from build123d import *

# Parameters (mm, degrees)
SKETCH1_R           = 6.35
BOSS_EXTRUDE1_DEPTH = 6.985
SKETCH3_R           = 8.382
BOSS_EXTRUDE2_DEPTH = 3.81
SKETCH5_R           = 2.5527
CUT_EXTRUDE2_DEPTH  = 56.328875207
SKETCH6_R           = 7.747
SKETCH6_R_2         = 6.096
CUT_EXTRUDE3_DEPTH  = 1.27


with BuildPart() as part:
    # Sketch1 → Boss-Extrude1 (new body)
    with BuildSketch(Plane.XY):
        with Locations((43.174261814, 8.550344032)):
            Circle(SKETCH1_R)
    extrude(amount=-BOSS_EXTRUDE1_DEPTH)

    # Sketch3 → Boss-Extrude2 (add)
    with BuildSketch(Plane.XY):
        with Locations(Location((43.174261814, 8.550344032, 0), (0, 0, 180))):
            Circle(SKETCH3_R)
    extrude(amount=BOSS_EXTRUDE2_DEPTH)

    # Sketch5 → Cut-Extrude2 (cut, through all)
    with BuildSketch(Plane(origin=(0, 0, -6.985), x_dir=(-1, 0, 0), z_dir=(0, 0, -1))):
        with Locations(Location((-43.174261814, 8.550344032, 0), (0, 0, 90))):
            Circle(SKETCH5_R)
    extrude(amount=-CUT_EXTRUDE2_DEPTH, mode=Mode.SUBTRACT)

    # Sketch6 → Cut-Extrude3 (cut)
    with BuildSketch(Plane.XY.offset(3.81)):
        with Locations((43.174261814, 8.550344032)):
            Circle(SKETCH6_R)
        with Locations((43.174261814, 8.550344032)):
            Circle(SKETCH6_R_2, mode=Mode.SUBTRACT)
    extrude(amount=-CUT_EXTRUDE3_DEPTH, mode=Mode.SUBTRACT)


solid = part.part
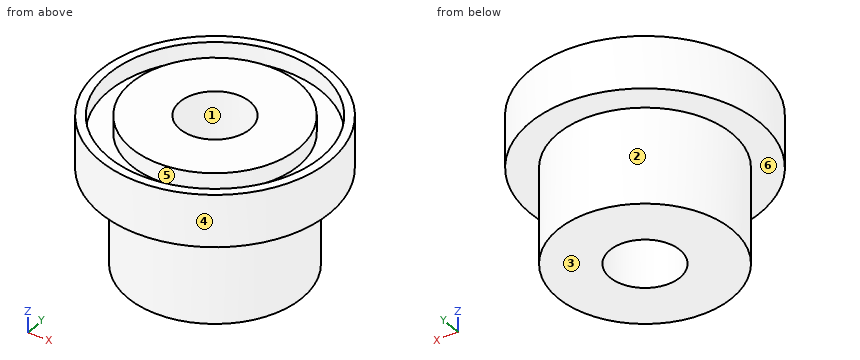
Geometry check sheet. Reference: the model listing, model coordinates, mm. Face numbers are marked on the shaded views. A direction names the side the tool comes from. Give positions to 0.01 mm unless a question says otherwise; leave off trailing zeros. Loops run counter-clockwise (first coordinate to the right, second up) from the corner with the lowest first, then second, coordinate; pieces in that order, holes last. Notation, with made-up numbers: M -38.75,59 L 6.25,59 A22 ccw 6.25,79 Z; hole C -35,21 d1. An arc over 180 degrees is marked long. Answer as a JSON object with one key per item and string values. Group by question number.
Item 1: Access from +Z, -Z, +X, -X, +Y, -Y to the whole of each face (thin tool, end or side, straight path). Record for the marked faces 4, 5 and 6.
Item 2: Sectioned sample at C-C on x = 47.75. Record the boundary of the cut face in (y, z) (1 decimal), plus the area to 3 significant figures.
Item 3: Mould release check, pull along Y, two halves, no side actions. Record for the marked faces 1, 2 and 3: pulls with the +Y half, pulls with the -Y half, needs draft (parallel to the pull), parting line crosses it, or undercut.
Item 4: Gauge pin test, flat ends, axial feed: pin 1 (2 mm diameter, centred on x = 40, z = -4, fed in from +Y); pin 2 (3 mm diameter, centred on x = 40.5, z = -2.5, fed in from -Y); pin 3 (2 mm diameter, centred on x = 42.5, y = 7.5, fed in from -Z). Record the tip position at first contact, or that the pin passes through.
Item 5: Sectioned sample at D-D on z = -0.5. Record the boundary of the cut face in (x, y).
Item 6: Sectioned sample at B-B on x = 42.5. Record the boundary of the cut face in (y, z) (1 decimal), plus the area to 3 significant figures.
Item 7: Material ranges on L1, parallel to X at y = 8.5, z = -3.5; L2, parallel to Y at x = 41, z = 2.75; L3, parallel to X at y = 6.25, z = -2, recorded low to high.
Item 8: Sectioned sample at A-A on y = 6.5. Record the boundary of the cut face in (x, z) (3 decimals), plus the area to 3 significant figures.
Findings below:
{
 "1": {"face 4": "+Z, -Z", "face 5": "+Z", "face 6": "-Z"},
 "2": {"outline": "M 1.5,0 L 4.1,0 L 4.1,-7 L 13,-7 L 13,0 L 15.6,0 L 15.6,3.8 L 14.8,3.8 L 14.8,2.5 L 12.6,2.5 L 12.6,3.8 L 4.5,3.8 L 4.5,2.5 L 2.3,2.5 L 2.3,3.8 L 1.5,3.8 Z", "area": "109 mm2"},
 "3": {"face 1": "undercut", "face 2": "parting line crosses it", "face 3": "needs draft"},
 "4": {"pin 1": "y = 14.52", "pin 2": "y = 2.31", "pin 3": "through"},
 "5": {"outline": "C 43.17,8.55 d12.7; hole C 43.17,8.55 d5.11"},
 "6": {"outline": "M 0.2,0 L 2.2,0 L 2.2,-7 L 6.1,-7 L 6.1,3.8 L 2.5,3.8 L 2.5,2.5 L 0.8,2.5 L 0.8,3.8 L 0.2,3.8 Z; M 11,-7 L 14.9,-7 L 14.9,0 L 16.9,0 L 16.9,3.8 L 16.3,3.8 L 16.3,2.5 L 14.6,2.5 L 14.6,3.8 L 11,3.8 Z", "area": "94.5 mm2"},
 "7": {"L1": "36.82 to 40.62, 45.73 to 49.52", "L2": "0.46 to 1.11, 2.86 to 7.21, 9.89 to 14.25, 15.99 to 16.65", "L3": "37.26 to 42.07, 44.28 to 49.09"},
 "8": {"outline": "M 35.047,0 L 37.164,0 L 37.164,-6.985 L 41.654,-6.985 L 41.654,3.81 L 37.433,3.81 L 37.433,2.54 L 35.704,2.54 L 35.704,3.81 L 35.047,3.81 Z; M 44.695,-6.985 L 49.184,-6.985 L 49.184,0 L 51.302,0 L 51.302,3.81 L 50.645,3.81 L 50.645,2.54 L 48.915,2.54 L 48.915,3.81 L 44.695,3.81 Z", "area": "109 mm2"}
}
